from build123d import *

# Parameters (mm, degrees)
F0_W     = 46.8
F0_H     = 2.5
F1_DEPTH = 49
F2_W     = 7.5
F2_H     = 1
F5_W     = 2.0469846204
F5_H     = 1.8061620649
F5_W_2   = 6.6439194979
F5_H_2   = 1.8455331939
F5_W_3   = 3.8363870533
F5_H_3   = 1.8061622977
F5_W_4   = 1.0836967267
F5_W_5   = 6.7777763455
F5_H_4   = 2
F5_W_6   = 1.8455331939
F5_H_5   = 3.3219597489
F6_DEPTH = 1.5


# Not quite as in the source:
# - a fillet or chamfer that OpenCascade refuses, or shapes differently, is made with other operations: its cross-section is extruded or revolved along the edge and cut away or added


with BuildPart() as f1:
    # F0 (on Front) → F1 (new body, symmetric)
    with BuildSketch(Plane.XZ):
        Polygon((25.3, -1.35), (25.3, 1.35), (23.3460554371, 1.35), (-23.4539445629, 1.35), (-25.3, 1.35), (-25.3, -1.35), align=None)
        with Locations((-0.0539445629, 2.6)):
            Rectangle(F0_W, F0_H)
    extrude(amount=F1_DEPTH, both=True)

    # F2 (on Front) → F3 (revolve, cut)
    with BuildSketch(Plane.XZ):
        with Locations((3.75, -0.85)):
            Rectangle(F2_W, F2_H)
    revolve(axis=Axis((0, 0, -0.85), (0, 0, -1)), mode=Mode.SUBTRACT)

    # F4: fillet of radius 5 on 1 edges, made by hand

    # F4_s1 → F4_t2 (revolve)
    with BuildSketch(Plane.XZ):
        with BuildLine():
            ThreePointArc((7.5, -1.35), (6.0811388301, -0.6065835097), (4.5, -0.35))
            Line((4.5, -0.35), (7.5, -0.35))
            Line((7.5, -0.35), (7.5, -1.35))
        make_face()
    revolve(axis=Axis((0, 0, -0.35), (0, 0, -1)))

    # F5 (on face) → F6 (join)
    with BuildSketch(Plane.XY.offset(3.85)):
        with BuildLine():
            Line((4.9241716042, 19.8006471619), (7.5009630335, 19.8006471619))
            add(Edge.make_bspline(
                [(7.5009630335, 19.8006471619), (7.9785124596, 19.5075781217), (8.9543671976, 18.9087022865), (7.3816458851, 17.3276064651), (4.7697273037, 17.0174018652), (3.1129348501, 16.8206328526)],
                knots=[0, 0, 0, 0, 0.2595051335, 0.5302892228, 1, 1, 1, 1], degree=3))
            Line((3.1129348501, 16.8206328526), (3.1129348501, 14.9474805221))
            Line((3.1129348501, 14.9474805221), (3.4767354373, 14.9474805221))
            add(Edge.make_bspline(
                [(3.4767354373, 14.9474805221), (4.5253869977, 15.1745288943), (5.5740385582, 15.4015772666), (6.6226901187, 15.6286256388)],
                knots=[0, 0, 0, 0, 3.2188490998, 3.2188490998, 3.2188490998, 3.2188490998], degree=3))
            Line((6.6226901187, 15.6286256388), (9.9595930205, 14.6069070324))
            Line((9.9595930205, 14.6069070324), (9.9595930205, 16.3097716868))
            Line((9.9595930205, 16.3097716868), (8.527294053, 16.7483240055))
            add(Edge.make_bspline(
                [(8.527294053, 16.7483240055), (9.0505266558, 16.9185557016), (10.2287332466, 17.301880642), (10.2116405832, 20.5168892904), (8.4127583201, 21.0586346497), (7.5009630335, 21.3332278654)],
                knots=[0, 0, 0, 0, 0.2826109345, 0.6363786658, 1, 1, 1, 1], degree=3))
            Line((7.5009630335, 21.3332278654), (3.3915922977, 21.3332278654))
            Line((3.3915922977, 21.3332278654), (3.3915922977, 18.2680701837))
            Line((3.3915922977, 18.2680701837), (4.9241716042, 18.2680701837))
            Line((4.9241716042, 18.2680701837), (4.9241716042, 19.8006471619))
        make_face()
        with BuildLine():
            Line((5.1796017215, 12.3080369085), (3.2213055529, 12.3080369085))
            Line((3.2213055529, 12.3080369085), (3.2213055529, 10.434884578))
            Line((3.2213055529, 10.434884578), (3.987595439, 10.434884578))
            add(Edge.make_bspline(
                [(7.0864924639, 10.434884578), (6.6226901187, 10.434884578), (5.6548767314, 10.434884578), (4.5585386607, 10.434884578), (3.987595439, 10.434884578)],
                knots=[0, 0, 0, 0, 0.4792270404, 1, 1, 1, 1], degree=3))
            add(Edge.make_bspline(
                [(7.0864924639, 10.434884578), (7.5009630335, 10.6619332607), (7.915433603, 10.8889819433), (8.3299041726, 11.116030626)],
                knots=[0, 0, 0, 0, 1.4177561906, 1.4177561906, 1.4177561906, 1.4177561906], degree=3))
            Line((8.3299041726, 11.116030626), (8.3299041726, 12.7337537706))
            add(Edge.make_bspline(
                [(5.1796017215, 12.3080369085), (5.4034691903, 12.3161910935), (5.946247887, 12.3359613528), (7.5456770883, 12.1555160266), (8.0916682054, 12.558094155), (8.3299041726, 12.7337537706)],
                knots=[0, 0, 0, 0, 0.2835019002, 0.6873655771, 1, 1, 1, 1], degree=3))
        make_face()
        with BuildLine():
            add(Edge.make_bspline(
                [(8.3299041726, 12.7337537706), (8.5748998169, 13.1310888877), (8.8198954612, 13.5284240047), (9.0648911056, 13.9257591218)],
                knots=[0, 0, 0, 0, 1.4003865712, 1.4003865712, 1.4003865712, 1.4003865712], degree=3))
            Line((8.3299041726, 12.7337537706), (8.3299041726, 11.116030626))
            Line((8.3299041726, 11.116030626), (8.3299041726, 9.4983074814))
            Line((8.3299041726, 9.4983074814), (9.0648911056, 9.4983074814))
            Line((9.0648911056, 9.4983074814), (9.9595930205, 9.4983074814))
            Line((9.9595930205, 9.4983074814), (9.9595930205, 13.9257591218))
            Line((9.9595930205, 13.9257591218), (9.0648911056, 13.9257591218))
        make_face()
        Polygon((8.1701891906, 8.3958084671), (7.0864924639, 8.3958084671), (5.1599194705, 7.1917017432), (5.1599194705, 5.3855396783), (7.0864924639, 6.5896464022), (8.1701891906, 6.5896464022), align=None)
        with Locations((4.1364271603, 6.2886207107)):
            Rectangle(F5_W, F5_H)
        Polygon((9.9595930205, 8.3958084671), (8.1701891906, 8.3958084671), (8.1701891906, 6.5896464022), (8.1701891906, 4.7834843373), (9.9595930205, 4.7834843373), align=None)
        Polygon((12.62538982, 4.7834843373), (9.9595930205, 4.7834843373), (8.1701891906, 4.7834843373), (8.1701891906, 2.9773220395), (12.62538982, 2.9773220395), align=None)
        with BuildLine():
            Line((8.1941955723, -4.5991633087), (9.157482069, -5.5624498054))
            add(Edge.make_bspline(
                [(9.157482069, -5.5624498054), (9.5487792454, -5.1790893624), (10.3709560961, -4.3735888355), (10.1809148183, -1.5911495575), (5.2901881268, -1.6214904462), (3.9387879664, -2.4019349259), (2.8327143669, -4.2152866088), (3.4405306211, -6.4549250287), (4.2493320025, -7.9388718891), (8.0091011439, -8.2673740434), (9.3225151381, -8.2281395815), (9.8799471743, -8.2114879042)],
                knots=[0, 0, 0, 0, 0.0955972377, 0.2008648172, 0.3547140558, 0.449658727, 0.5522106806, 0.6629402054, 0.7557007662, 0.8963158456, 1, 1, 1, 1], degree=3))
            Line((9.8799471743, -8.2114879042), (9.8799471743, -6.2849144451))
            Line((9.8799471743, -6.2849144451), (9.639125783, -6.2849144451))
            Line((9.639125783, -6.2849144451), (5.7859793305, -6.2849144451))
            add(Edge.make_bspline(
                [(5.7859793305, -6.2849144451), (5.3373815573, -6.0824238319), (4.5029895973, -5.7057912452), (4.6151304787, -4.5054927526), (5.5221677114, -3.357555761), (8.2143823017, -3.3336799886), (8.8829973904, -4.2841414137), (8.4141443171, -4.4985702665), (8.1941955723, -4.5991633087)],
                knots=[0, 0, 0, 0, 0.1746613826, 0.3248702113, 0.5034996406, 0.7468657523, 0.8812494506, 1, 1, 1, 1], degree=3))
        make_face()
        with Locations((6.4990330953, -10.5825328623)):
            Rectangle(F5_W_2, F5_H_2)
        with BuildLine():
            Line((5.094458349, -12.8092374653), (3.2213055529, -12.8092374653))
            Line((3.2213055529, -12.8092374653), (3.2213055529, -19.3652724847))
            Line((3.2213055529, -19.3652724847), (4.753885325, -19.3652724847))
            Line((4.753885325, -19.3652724847), (4.753885325, -15.7041111961))
            Line((4.753885325, -15.7041111961), (7.393327076, -15.7041111961))
            add(Edge.make_bspline(
                [(7.393327076, -15.7041111961), (7.7280745564, -15.8906025071), (8.6028551514, -16.3779518959), (8.4340893146, -18.2776591394), (8.3299041726, -19.4504158571)],
                knots=[0, 0, 0, 0, 0.3826645017, 1, 1, 1, 1], degree=3))
            Line((8.3299041726, -19.4504158571), (9.777339641, -19.4504158571))
            add(Edge.make_bspline(
                [(9.777339641, -19.4504158571), (9.916282957, -18.4574178062), (10.1622140126, -16.6998013476), (9.7862090494, -14.9229979542), (8.1515194, -13.6961261057), (6.2020376655, -13.8364032587), (5.094458349, -13.9161003754)],
                knots=[0, 0, 0, 0, 0.2773941316, 0.4909903808, 0.7108110755, 1, 1, 1, 1], degree=3))
            Line((5.094458349, -13.9161003754), (5.094458349, -12.8092374653))
        make_face()
        Polygon((-8.0897600321, 22.7236154125), (-7.0060633053, 22.7236154125), (-7.0060633053, 24.5297774774), (-8.0897600321, 24.5297774774), (-10.0163330255, 23.3256707535), (-12.0633176458, 23.3256707535), (-12.0633176458, 21.5195086886), (-10.0163330255, 21.5195086886), align=None)
        Polygon((-7.0060633053, 20.9174533476), (-5.2166594755, 20.9174533476), (-5.2166594755, 24.5297774774), (-7.0060633053, 24.5297774774), (-7.0060633053, 22.7236154125), align=None)
        Polygon((-7.0060633053, 19.1112910499), (-2.550862676, 19.1112910499), (-2.550862676, 20.9174533476), (-5.2166594755, 20.9174533476), (-7.0060633053, 20.9174533476), align=None)
        with Locations((-7.1348530021, 17.1245136399)):
            Rectangle(F5_W_3, F5_H_3)
        Polygon((-9.9878371693, 8.1643839367), (-8.0612641759, 9.3684906606), (-8.0612641759, 11.1746527255), (-9.9878371693, 9.9705460016), (-12.0348217897, 9.9705460016), (-12.0348217897, 8.1643839367), align=None)
        with Locations((-7.5194158126, 10.271571693)):
            Rectangle(F5_W_4, F5_H)
        Polygon((-6.9775674492, 9.3684906606), (-6.9775674492, 7.5623285957), (-5.1881636194, 7.5623285957), (-5.1881636194, 11.1746527255), (-6.9775674492, 11.1746527255), align=None)
        Polygon((-6.9775674492, 5.7561662979), (-2.5223668199, 5.7561662979), (-2.5223668199, 7.5623285957), (-5.1881636194, 7.5623285957), (-6.9775674492, 7.5623285957), align=None)
        with Locations((-7.106357146, 3.769388888)):
            Rectangle(F5_W_3, F5_H_3)
        with Locations((-8.5770517921, -3.2183615263)):
            Rectangle(F5_W_5, F5_H_4)
        with Locations((-8.560137578, -6.9900213829)):
            Rectangle(F5_W_6, F5_H_5)
        Polygon((-7.969349802, -15.0853700369), (-6.8856530753, -15.0853700369), (-6.8856530753, -13.279207972), (-7.969349802, -13.279207972), (-9.8959227954, -14.4833146959), (-11.9429074158, -14.4833146959), (-11.9429074158, -16.2894767608), (-9.8959227954, -16.2894767608), align=None)
        Polygon((-6.8856530753, -15.0853700369), (-6.8856530753, -16.8915321018), (-5.0962492455, -16.8915321018), (-5.0962492455, -13.279207972), (-6.8856530753, -13.279207972), align=None)
        Polygon((-6.8856530753, -18.6976943995), (-2.430452446, -18.6976943995), (-2.430452446, -16.8915321018), (-5.0962492455, -16.8915321018), (-6.8856530753, -16.8915321018), align=None)
        with Locations((-7.0144427721, -20.6844718094)):
            Rectangle(F5_W_3, F5_H_3)
    extrude(amount=F6_DEPTH)


solid = f1.part
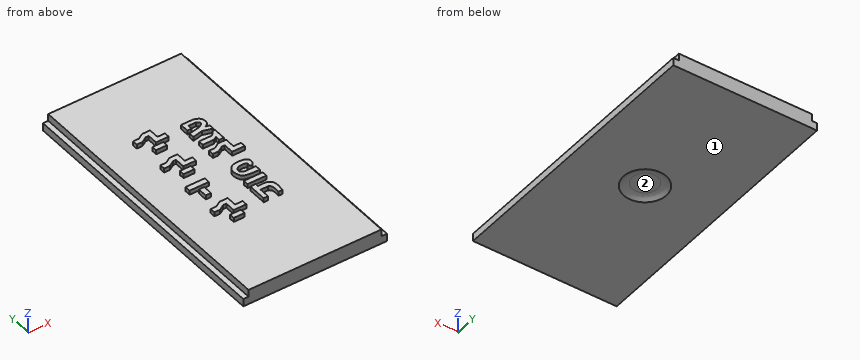
Work out the finished part from the listing and answer in its coordinate system (mm). Face numbers are marked on the shaded views. Round coordinates to 2 decimals unless told otherwise and drop trailing zeros. Loops run counter-clockwise (first coordinate to the right, second up) from the corner with the lowest first, then second, coordinate; pieces in that order, holes last. Notation, with made-up numbers: (62, -23) - (81, -23) arc R23 cw to (81, -6) - close; hole circle Ø1 at (-8, 66). An arc over 180 degrees is marked (long way). Use one line per item in the form item = value. Start each with the question number.
(1) Flat-ended cylindrical pins translate along their axes: P1, Ø0.7, axis at x = -7.5, z = 4.5, coming from the -Y side; P2, Ø1.6, axis at x = 24, y = 4.5, coming from the +Z side; P3, Ø3, axis at y = -7, z = 3, coming from the -X side. Find the tip coordinate at first contact, or state that the pin passes through.
(2) Find section C-C on x = 19. Determine the outline of the cut face in (y, z).
(3) Consider line 1 (Y direction, x = -5, z = 4.75); line 2 (Z direction, x = -3, y = -31.5); line 3 (X direction, y = 40.5, z = 3.25). Determine where each line is inside the solid, lowest interval first.
(4) Find section A-A on x = 11.5. Determine the outline of the cut face in (y, z).
(5) Find section B-B on y = 36. Determine the outline of the cut face in (x, z), and give its area (3 significant figures).
(6) Determine the mould class of the marked faces 1 and 2 for opening direction Y: +Y half, -Y half, draft (parallel to the pull), parting line (faces both ways), or undercut.
Answer list:
q1.P1 = -21.59
q1.P2 = 3.85
q1.P3 = -23.45
q2.outline = (-49, -1.35) - (49, -1.35) - (49, 3.85) - (-49, 3.85) - close
q3.line_1 = -18.7 to -16.89, 5.76 to 7.56, 19.11 to 20.92
q3.line_2 = -1.35 to 3.85
q3.line_3 = -23.45 to 23.35
q4.outline = (-49, -1.35) - (49, -1.35) - (49, 3.85) - (4.78, 3.85) - (4.78, 5.35) - (2.98, 5.35) - (2.98, 3.85) - (-49, 3.85) - close
q5.outline = (-25.3, -1.35) - (25.3, -1.35) - (25.3, 1.35) - (23.35, 1.35) - (23.35, 3.85) - (-23.45, 3.85) - (-23.45, 1.35) - (-25.3, 1.35) - close
q5.area = 254 mm^2
q6.face_1 = draft
q6.face_2 = undercut
